Verification items for this drawing (mm, ordinates from the low corner). A direction names the side the tool comes from. Round coordinates to 2 decimals unless told otherwise and drop trailing zeros. Write each loop counter-clockwise with the first axis right and the second up, starting at its lowest first coordinate (ties: lowest second). Pieces come first, ordered by that corner, then holes.
Item 1: Cross-section at D-D (x = 13). Enter the section's corners in (y, z).
Item 2: Access from +Z, -Z, +X, -X, +Y, -Y to the whole of each face (thin tool, end or side, straight path). Record for the marked faces 5 and 6.
Item 3: Cross-section at C-C (x = 10.5). Enter the section's corners in (y, z).
Item 4: Cross-section at B-B (y = 11.75). Enter the section's corners in (x, z), then the cut area to 3 significant figures.
Item 5: Depth check by flat-ended pin: P1, Ø2, axis at x = 15, y = 4.5, coming from the -Z side. Enter the tip coordinate at first touch or a pass-through.
Item 6: Scan lines: probe 1 along X at (y, z) = (13, 6.75); probe 2 along X at (y, z) = (5.75, 4.25); probe 3 along Z at (x, y) = (12.75, 10.75). Record each from-to range of solid material in increasing order.
Item 7: Draft check along Y on the marked faces 1, 2, 3 and 4. Enter one of: pulls with the +Y half, pulls with the -Y half, needs draft (parallel to the pull), parting line crosses it, or undercut.
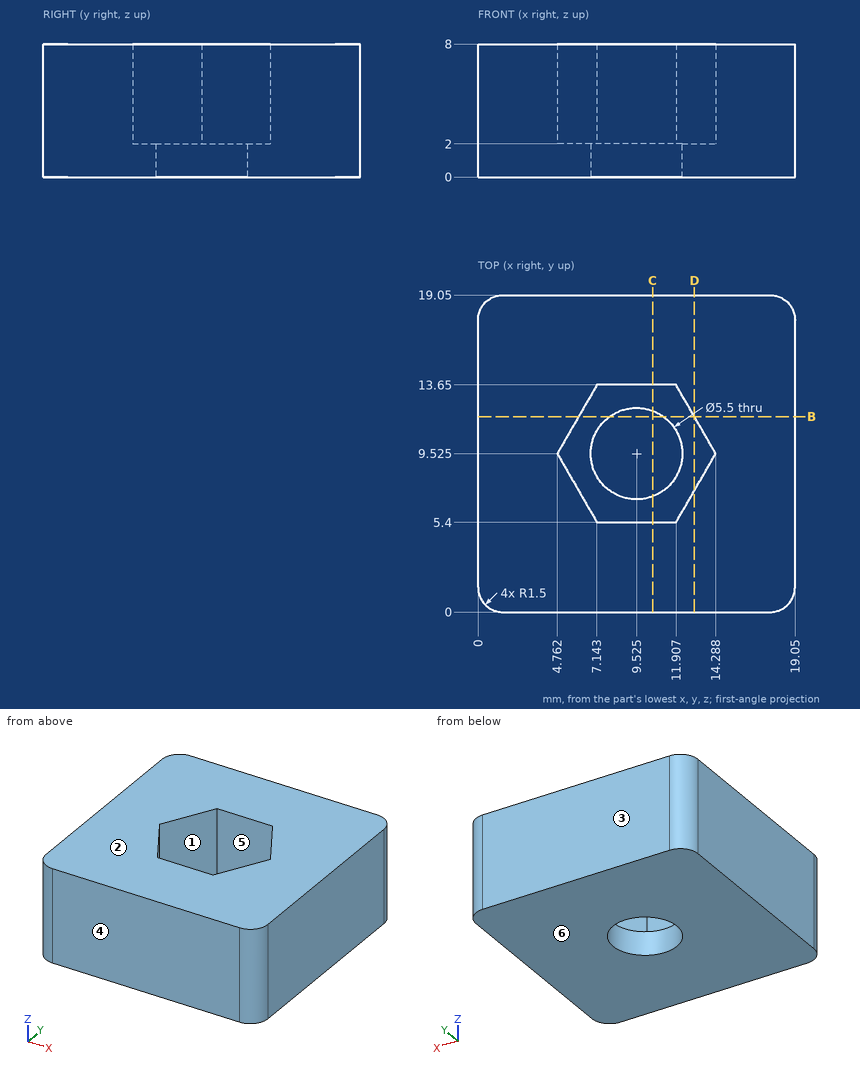
Resolved:
1. outline: (0, 0) - (19.05, 0) - (19.05, 8) - (11.76, 8) - (11.76, 2) - (7.29, 2) - (7.29, 8) - (0, 8) - close
2. face 5: +Z
2. face 6: -Z, +X, -X, +Y, -Y
3. outline: (0, 0) - (6.95, 0) - (6.95, 2) - (5.4, 2) - (5.4, 8) - (0, 8) - close; (12.1, 0) - (19.05, 0) - (19.05, 8) - (13.65, 8) - (13.65, 2) - (12.1, 2) - close
4. outline: (0, 0) - (7.91, 0) - (7.91, 2) - (6.05, 2) - (6.05, 8) - (0, 8) - close; (11.14, 0) - (19.05, 0) - (19.05, 8) - (13, 8) - (13, 2) - (11.14, 2) - close
4. area: 104 mm2
5. P1: stops at z = 0
6. probe 1: x = 0 to 6.77, 12.28 to 19.05
6. probe 2: x = 0 to 6.94, 12.11 to 19.05
6. probe 3: z = 0 to 2
7. face 1: undercut
7. face 2: needs draft
7. face 3: pulls with the +Y half
7. face 4: pulls with the -Y half
